Read the model definition and answer for the solid it produces. Units are mm, in the model's axes. A direction names the side the tool comes from. Coordinates: 2 decimals unless noted, no trailing zeros. Write each loop counter-clockwise with the first axis right and the second up, starting at its lowest first coordinate (ties: lowest second). Pieces come first, ordered by that corner, then holes. Notation, with made-up numbers: (80.5, -17.75) -> (117.5, -17.75) arc R11 ccw to (117.5, 3.25) -> close; hole circle Ø1 at (13, 54.5). An arc over 180 degrees is marked (long way). Write item = value, one per line. Start each with the question number.
1) For a pull along Z with two mould halves and no side action, classify faces 4 (the face through (15.273, 0.986, 23.297)), 5 (the face through (4, 80, 49)), 6 (the face through (-5.27, 0.99, -2.51)) as released by +Z, released by -Z, zero draft, split by the parting line, or undercut.
2) Section C-C (x = -64.5) is taken. Determine the outline of the cut face in (y, z), plus the area to 4 significant figures.
3) Section B-B (y = 85.5) is taken. Determine the outline of the cut face in (x, z), plus the area to 3 significant figures.
4) Section A-A (y = 28.5) is taken. Determine the outline of the cut face in (x, z).
5) Find the intervals of material crossed by line 1 along Z through (x, y) = (-1, 9); line 2 along Z through (x, y) = (-84.7, 90); line 3 along Y through (x, z) = (-84.45, 0), in increasing order. Write a range as from..to.
6) Section D-D (y = 67) is taken. Determine the outline of the cut face in (x, z), plus the area to 3 significant figures.
7) A tool of negligible diameter and unlimited length cuts with its end or side. For faces 1 (the face through (90.5, 39, 29)), 2 (the face through (88, 41, 1)), 3 (the face through (15.58, 0.99, 4.84)), from which of +Z, -Z, +X, -X, +Y, -Y can it reach the whole face along a straight path? Write none if from no direction.
8) Flat-ended cylindrical pins translate along their axes: pin 1 Ø1.2 at (x, y) = (-84.5, 49) entering from -Z; pin 2 Ø1.5 at (x, z) = (42.5, -15) entering from -Y; pin 3 Ø12 at (x, z) = (22.5, 9) entering from -Y; pin 4 Ø10 at (y, z) = (32.5, 29) entering from -X. Find the tip coordinate at first contact, or state that the pin passes through.
from build123d import *

# Parameters (mm, degrees)
SKETCH1_W           = 173
SKETCH1_H           = 100
BOSS_EXTRUDE1_DEPTH = 80
SHELL2_T            = -2.5
SKETCH3_W           = 3
SKETCH3_H           = 10
BOSS_EXTRUDE2_DEPTH = 95
CHAMFER1_SIZE       = 2
MOVE_FACE1_BY       = 0.5
MOVE_FACE2_BY       = 0.5
SKETCH4_R           = 1.5
CUT_EXTRUDE1_DEPTH  = 209.724699066
CUT_EXTRUDE3_DEPTH  = 2
SKETCH6_W           = 15
SKETCH6_H           = 25
CUT_EXTRUDE4_DEPTH  = 207.157706623


# Read off the part's stored shape, not the designer's step: Cut-Extrude3
with BuildPart() as part:
    # Sketch1 → Boss-Extrude1 (new body)
    with BuildSketch(Plane(origin=(0, 0, 0), x_dir=(1, 0, 0), z_dir=(0, 1, 0))):
        with Locations((4, 0)):
            Rectangle(SKETCH1_W, SKETCH1_H)
    extrude(amount=BOSS_EXTRUDE1_DEPTH)

    # Shell2
    shell2_openings = [part.faces().sort_by_distance(p)[0] for p in [
        (4, 80, 0),
    ]]
    offset(amount=SHELL2_T, openings=shell2_openings, kind=Kind.INTERSECTION)

    # Sketch3 → Boss-Extrude2 (add)
    with BuildSketch(Plane.XZ):
        with Locations((-84, 0)):
            Rectangle(SKETCH3_W, SKETCH3_H)
        with Locations((92, 0)):
            Rectangle(SKETCH3_W, SKETCH3_H)
    extrude(amount=-BOSS_EXTRUDE2_DEPTH)

    # Chamfer1
    chamfer1_edges = [part.edges().sort_by_distance(p)[0] for p in [
        (90.5, 40, 5),
        (90.5, 40, -5),
        (-82.5, 40, -5),
        (-82.5, 40, 5),
        (92, 95, 5),
        (92, 95, -5),
        (-84, 95, -5),
        (-84, 95, 5),
    ]]
    chamfer(chamfer1_edges, length=CHAMFER1_SIZE)

    # Move Face1: a face moved inward by 0.5
    extrude(part.faces().sort_by_distance((-82.5, 87.312785388, 0))[0], amount=MOVE_FACE1_BY, dir=(-1, 0, 0), mode=Mode.SUBTRACT)

    # Move Face2: a face moved inward by 0.5
    extrude(part.faces().sort_by_distance((90.5, 87.312785388, 0))[0], amount=MOVE_FACE2_BY, dir=(1, 0, 0), mode=Mode.SUBTRACT)

    # Sketch4 → Cut-Extrude1 (cut, through all)
    with BuildSketch(Plane.ZY.offset(85.5)):
        with Locations((0, 90)):
            Circle(SKETCH4_R)
    extrude(amount=-CUT_EXTRUDE1_DEPTH, mode=Mode.SUBTRACT)

    # Cut-Extrude3 outline → Cut-Extrude3 (cut)
    with BuildSketch(Plane(origin=(0, 0, 0), x_dir=(1, 0, 0), z_dir=(0, 1, 0))):
        Polygon((80.5, 2.857864376), (80.5, 40), (-72.5, 40), (-72.5, 2.857864376), (-75.357864376, 0), (-72.5, -2.857864376), (-72.5, -40), (80.5, -40), (80.5, -2.857864376), (83.357864376, 0), align=None)
        Polygon((7.417714413, -17.552090263), (12.749188197, -19.378229604), (-23.808346413, 25.027697518), (3.280599797, 4.287723077), (-3.809085344, 7.144760372), (11.640079291, -13.383581677), (12.749188197, -10.769740582), (15.558903364, -13.383581677), (11.640079291, -2.041689211), (19.62402318, -7.712635444), (21.716364262, -22.427069466), (15.060881541, -16.235561356), (14.410666008, -17.767926727), (22.911987737, -28.883436233), align=None, mode=Mode.SUBTRACT)
    extrude(amount=CUT_EXTRUDE3_DEPTH, mode=Mode.SUBTRACT)

    # Sketch6 → Cut-Extrude4 (cut, through all)
    with BuildSketch(Plane.ZY.offset(82.5)):
        with Locations((22.5, 67.5)):
            Rectangle(SKETCH6_W, SKETCH6_H)
    extrude(amount=-CUT_EXTRUDE4_DEPTH, mode=Mode.SUBTRACT)


solid = part.part
Answer key:
q1.face_4 = undercut
q1.face_5 = zero draft
q1.face_6 = undercut
q2.outline = (0, -50) -> (80, -50) -> (80, -47.5) -> (2.5, -47.5) -> (2.5, 47.5) -> (80, 47.5) -> (80, 50) -> (0, 50) -> (0, 40) -> (2, 40) -> (2, -40) -> (0, -40) -> close
q2.area = 477.5 mm^2
q3.outline = (-85.5, -5) -> (-83, -5) -> (-83, 5) -> (-85.5, 5) -> close; (91, -5) -> (93.5, -5) -> (93.5, 5) -> (91, 5) -> close
q3.area = 50.0 mm^2
q4.outline = (-85.5, -5) -> (-84.5, -5) -> (-82.5, -7) -> (-82.5, -50) -> (90.5, -50) -> (90.5, -7) -> (92.5, -5) -> (93.5, -5) -> (93.5, 5) -> (92.5, 5) -> (90.5, 7) -> (90.5, 50) -> (-82.5, 50) -> (-82.5, 7) -> (-84.5, 5) -> (-85.5, 5) -> close; hole (-80, -47.5) -> (88, -47.5) -> (88, 47.5) -> (-80, 47.5) -> close
q5.line_1 = -50..-47.5, 47.5..50
q5.line_2 = -5..-1.5, 1.5..5
q5.line_3 = 0..88.5, 91.5..95
q6.outline = (-85.5, -5) -> (-84.5, -5) -> (-82.5, -7) -> (-82.5, -50) -> (90.5, -50) -> (90.5, -7) -> (92.5, -5) -> (93.5, -5) -> (93.5, 5) -> (92.5, 5) -> (90.5, 7) -> (90.5, 15) -> (88, 15) -> (88, -47.5) -> (-80, -47.5) -> (-80, 15) -> (-82.5, 15) -> (-82.5, 7) -> (-84.5, 5) -> (-85.5, 5) -> close; (-82.5, 30) -> (-80, 30) -> (-80, 47.5) -> (88, 47.5) -> (88, 30) -> (90.5, 30) -> (90.5, 50) -> (-82.5, 50) -> close
q6.area = 1,330 mm^2
q7.face_1 = +Z, +X, +Y, -Y
q7.face_2 = +Y
q7.face_3 = -Y
q8.pin_1 = -5.6
q8.pin_2 = 2
q8.pin_3 = 0
q8.pin_4 = -82.5
